Model file for the job. Use its own axes, mm. Face numbers are marked on the shaded views. A direction names the side the tool comes from. Round coordinates to 2 decimals unless told otherwise and drop trailing zeros. Order: outer loops, then holes, each group sorted by start corner. A loop starts at its lowest first (then second) coordinate and runs counter-clockwise, first axis right, second up. Notation, with made-up numbers: (53, -19) -> (81, -19) arc R9 ccw to (81, -4) -> close; hole circle Ø11 at (-36.75, -28). An arc over 180 degrees is marked (long way). Use CSV: the item, a comma, the result in double quotes.
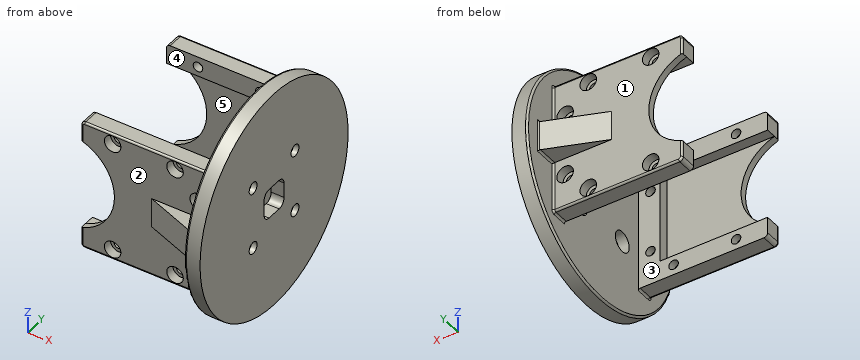
```python
from build123d import *

# Parameters (mm, degrees)
SKETCH1_R           = 1.3
BOSS_EXTRUDE1_DEPTH = 2.8
SKETCH2_R           = 1.3
BOSS_EXTRUDE2_DEPTH = 1.8
SKETCH3_R           = 2.25
CUT_EXTRUDE1_DEPTH  = 2.5
SKETCH4_W           = 35.6
SKETCH4_H           = 4.6
BOSS_EXTRUDE3_DEPTH = 5
SKETCH5_W           = 4.2
SKETCH5_H           = 35.6
BOSS_EXTRUDE4_DEPTH = 15
FILLET1_R           = 1
SKETCH6_R           = 1.6
CUT_EXTRUDE2_DEPTH  = 40.396155741
SKETCH7_R           = 2.8
CUT_EXTRUDE3_DEPTH  = 2.7
CUT_EXTRUDE4_DEPTH  = 3.5
SKETCH9_R           = 30
SKETCH9_W           = 35.6
SKETCH9_H           = 39.2
BOSS_EXTRUDE5_DEPTH = 4.2
BOSS_EXTRUDE6_DEPTH = 4
FILLET2_R           = 0.5
FILLET3_R           = 0.5


with BuildPart() as part:
    # Sketch1 → Boss-Extrude1 (new body)
    with BuildSketch(Plane(origin=(0, 0, 0), x_dir=(1, 0, 0), z_dir=(0, 1, 0))):
        Polygon((33.2, 12.4), (33.2, -12.4), (3.903844259, -12.4), (3.903844259, -17.8), (38.3, -17.8), (38.3, 17.8), (3.903844259, 17.8), (3.903844259, 12.4), align=None)
        with Locations((12.5, 15)):
            Circle(SKETCH1_R, mode=Mode.SUBTRACT)
        with Locations((29.5, 15)):
            Circle(SKETCH1_R, mode=Mode.SUBTRACT)
        with Locations((29.5, -15)):
            Circle(SKETCH1_R, mode=Mode.SUBTRACT)
        with Locations((12.5, -15)):
            Circle(SKETCH1_R, mode=Mode.SUBTRACT)
        with Locations((35.8, -8.5)):
            Circle(SKETCH1_R, mode=Mode.SUBTRACT)
        with Locations((35.8, 8.5)):
            Circle(SKETCH1_R, mode=Mode.SUBTRACT)
    extrude(amount=BOSS_EXTRUDE1_DEPTH)

    # Sketch2 → Boss-Extrude2 (add)
    with BuildSketch(Plane(origin=(0, 2.8, 0), x_dir=(1, 0, 0), z_dir=(0, 1, 0))):
        with BuildLine():
            Line((3.903844259, -12.4), (3.903844259, -17.8))
            Line((3.903844259, -17.8), (38.3, -17.8))
            Line((38.3, -17.8), (38.3, 17.8))
            Line((38.3, 17.8), (3.903844259, 17.8))
            Line((3.903844259, 17.8), (3.903844259, 12.4))
            ThreePointArc((3.903844259, 12.4), (13, 0), (3.903844259, -12.4))
        make_face()
        with Locations((12.5, -15)):
            Circle(SKETCH2_R, mode=Mode.SUBTRACT)
        with Locations((29.5, -15)):
            Circle(SKETCH2_R, mode=Mode.SUBTRACT)
        with Locations((35.8, -8.5)):
            Circle(SKETCH2_R, mode=Mode.SUBTRACT)
        with Locations((35.8, 8.5)):
            Circle(SKETCH2_R, mode=Mode.SUBTRACT)
        with Locations((29.5, 15)):
            Circle(SKETCH2_R, mode=Mode.SUBTRACT)
        with Locations((12.5, 15)):
            Circle(SKETCH2_R, mode=Mode.SUBTRACT)
    extrude(amount=BOSS_EXTRUDE2_DEPTH)

    # Sketch3 → Cut-Extrude1 (cut)
    with BuildSketch(Plane(origin=(0, 4.6, 0), x_dir=(1, 0, 0), z_dir=(0, 1, 0))):
        with Locations((12.5, 15)):
            Circle(SKETCH3_R)
        with Locations((29.5, 15)):
            Circle(SKETCH3_R)
        with Locations((35.8, 8.5)):
            Circle(SKETCH3_R)
        with Locations((35.8, -8.5)):
            Circle(SKETCH3_R)
        with Locations((29.5, -15)):
            Circle(SKETCH3_R)
        with Locations((12.5, -15)):
            Circle(SKETCH3_R)
    extrude(amount=-CUT_EXTRUDE1_DEPTH, mode=Mode.SUBTRACT)

    # Sketch4 → Boss-Extrude3 (add)
    with BuildSketch(Plane(origin=(38.3, 0, 0), x_dir=(0, 0, -1), z_dir=(1, 0, 0))):
        with Locations((0, 2.3)):
            Rectangle(SKETCH4_W, SKETCH4_H)
    extrude(amount=BOSS_EXTRUDE3_DEPTH)

    # Sketch5 → Boss-Extrude4 (add)
    with BuildSketch(Plane.XZ):
        with Locations((41.2, 0)):
            Rectangle(SKETCH5_W, SKETCH5_H)
    extrude(amount=BOSS_EXTRUDE4_DEPTH)

    # Mirror1: part across plane


with BuildPart() as part_1:
    add(part.part)
    add(part.part.mirror(Plane.ZX.offset(-15)))

    # Fillet1
    fillet1_edges = [part_1.edges().sort_by_distance(p)[0] for p in [
        (3.903844259, 2.3, -17.8),
        (3.903844259, 2.3, 17.8),
        (3.903844259, -32.3, 17.8),
        (3.903844259, -32.3, -17.8),
    ]]
    fillet(fillet1_edges, radius=FILLET1_R)

    # Sketch6 → Cut-Extrude2 (cut, through all)
    with BuildSketch(Plane(origin=(43.3, 0, 0), x_dir=(0, 0, -1), z_dir=(1, 0, 0))):
        with Locations((8.485281374, -23.485281374)):
            Circle(SKETCH6_R)
        with Locations((-8.485281374, -23.485281374)):
            Circle(SKETCH6_R)
        with Locations((-8.485281374, -6.514718626)):
            Circle(SKETCH6_R)
        with Locations((8.485281374, -6.514718626)):
            Circle(SKETCH6_R)
    extrude(amount=-CUT_EXTRUDE2_DEPTH, mode=Mode.SUBTRACT)

    # Sketch7 → Cut-Extrude3 (cut)
    with BuildSketch(Plane.ZY.offset(-39.1)):
        with Locations((-8.485281374, -6.514718626)):
            Circle(SKETCH7_R)
        with Locations((8.485281374, -6.514718626)):
            Circle(SKETCH7_R)
        with Locations((-8.485281374, -23.485281374)):
            Circle(SKETCH7_R)
        with Locations((8.485281374, -23.485281374)):
            Circle(SKETCH7_R)
    extrude(amount=-CUT_EXTRUDE3_DEPTH, mode=Mode.SUBTRACT)

    # Sketch8 → Cut-Extrude4 (cut)
    with BuildSketch(Plane(origin=(43.3, 0, 0), x_dir=(0, 0, -1), z_dir=(1, 0, 0))):
        with BuildLine():
            Line((-2.05, -19.05), (2.05, -19.05))
            ThreePointArc((2.05, -19.05), (3.464213562, -18.464213562), (4.05, -17.05))
            Line((4.05, -17.05), (4.05, -12.95))
            ThreePointArc((4.05, -12.95), (3.464213562, -11.535786438), (2.05, -10.95))
            Line((2.05, -10.95), (-2.05, -10.95))
            ThreePointArc((-2.05, -10.95), (-3.464213562, -11.535786438), (-4.05, -12.95))
            Line((-4.05, -12.95), (-4.05, -17.05))
            ThreePointArc((-4.05, -17.05), (-3.464213562, -18.464213562), (-2.05, -19.05))
        make_face()
    extrude(amount=-CUT_EXTRUDE4_DEPTH, mode=Mode.SUBTRACT)

    # Sketch9 → Boss-Extrude5 (add)
    with BuildSketch(Plane(origin=(43.3, 0, 0), x_dir=(0, 0, -1), z_dir=(1, 0, 0))):
        with Locations((0, -15)):
            Circle(SKETCH9_R)
        with Locations((0, -15)):
            Rectangle(SKETCH9_W, SKETCH9_H, mode=Mode.SUBTRACT)
    extrude(amount=-BOSS_EXTRUDE5_DEPTH)

    # Sketch10 → Boss-Extrude6 (add, symmetric)
    with BuildSketch(Plane.XY):
        Polygon((39.1, 10.6), (39.1, 4.6), (23.1, 4.6), align=None)
    boss_extrude6 = extrude(amount=BOSS_EXTRUDE6_DEPTH, both=True)

    # Mirror2: Boss-Extrude6 across plane
    add(boss_extrude6.mirror(Plane(origin=(0, -15, 0), x_dir=(0, 0, 1), z_dir=(0, -1, 0))))

    # Fillet2
    fillet2_edges = [part_1.edges().sort_by_distance(p)[0] for p in [
        (39.1, -15, 30),
    ]]
    fillet(fillet2_edges, radius=FILLET2_R)

    # Fillet3
    fillet3_edges = [part_1.edges().sort_by_distance(p)[0] for p in [
        (3.903844259, -34.6, 14.6),
        (3.903844259, 4.6, -14.6),
        (22.00192213, 4.6, 17.8),
        (4.196737478, 4.6, 17.507106781),
        (4.196737478, 4.6, -17.507106781),
        (3.903844259, -34.6, -14.6),
        (22.00192213, -34.6, 17.8),
        (4.196737478, -34.6, 17.507106781),
        (4.196737478, -34.6, -17.507106781),
        (22.00192213, -34.6, -17.8),
        (22.00192213, 4.6, -17.8),
        (39.1, -32.3, 17.8),
        (39.1, 2.3, 17.8),
        (39.1, -34.6, -10.9),
        (39.1, 2.3, -17.8),
        (39.1, -32.3, -17.8),
        (39.1, 4.6, 10.9),
        (39.1, 4.6, -10.9),
        (39.1, 10.6, 0),
        (39.1, 7.6, -4),
        (39.1, 7.6, 4),
        (39.1, -34.6, 10.9),
        (39.1, -37.6, 4),
        (39.1, -40.6, 0),
        (39.1, -37.6, -4),
        (3.903844259, 4.6, 14.6),
    ]]
    fillet(fillet3_edges, radius=FILLET3_R)


solid = part_1.part
```
Q1. Probe line 1 along X through (y, z) = (3, -15); line 2 along Z through (x, y) = (12.5, -31.2); line 3 along Y through (x, z) = (32, 17). List the from-to ranges inside material, lowest first.
From the geometry:
line 1,"x = 3.9 to 10.25, 14.75 to 27.25, 31.75 to 43.3"
line 2,"z = -17.8 to -16.3, -13.7 to -12.4, 12.4 to 13.7, 16.3 to 17.8"
line 3,"y = -34.6 to -30, 0 to 4.6"
Q2. Which spindle directions (+Z, -Z, +X, -X, +Y, -Y) get a long thin tool onto all of the face, cutting with end or side? Do the marked faces 1, 2 and 3. Say none if no direction does.
From the geometry:
face 1,"-X, +Y"
face 2,"-X, -Y"
face 3,"+Z, -Z, -X"
Q3. Pin check, flat tips, straight feed: pin 1 (1.4 mm diameter, centred on y = -31, z = 2, fed in from -X); pin 2 (1.7 mm diameter, centred on x = 30, y = 8.5, fed in from +Z); pin 3 (7 mm diameter, centred on x = 35.8, z = 8.5, fed in from -Y); pin 4 (2 mm diameter, centred on x = 29.5, y = 3, fed in from -Z). Stop position of each tip, or through.
From the geometry:
pin 1,"stops at x = 33.2"
pin 2,"passes through"
pin 3,"stops at y = -43.8"
pin 4,"stops at z = -17.8"
Q4. Cut at C-C (y = -15). Give the cut face in (x, z).
From the geometry:
outline,"(39.1, -29.5) arc R0.5 ccw to (39.6, -30) -> (43.3, -30) -> (43.3, -4.05) -> (39.8, -4.05) -> (39.8, 4.05) -> (43.3, 4.05) -> (43.3, 30) -> (39.6, 30) arc R0.5 ccw to (39.1, 29.5) -> close"
Q5. Mould opens along Z. For the marked faces 4 and 5 say: +Z half, -Z half, draft (parallel to the pull), parting line (faces both ways), or undercut.
From the geometry:
face 4,"draft"
face 5,"undercut"
Q6. Cut at A-A (x = 17). Give the cut face in (y, z).
From the geometry:
outline,"(-34.6, -17.3) arc R0.5 ccw to (-34.1, -17.8) -> (-30, -17.8) -> (-30, -12.4) -> (-32.8, -12.4) -> (-32.8, 12.4) -> (-30, 12.4) -> (-30, 17.8) -> (-34.1, 17.8) arc R0.5 ccw to (-34.6, 17.3) -> close; (0, -17.8) -> (4.1, -17.8) arc R0.5 ccw to (4.6, -17.3) -> (4.6, 17.3) arc R0.5 ccw to (4.1, 17.8) -> (0, 17.8) -> (0, 12.4) -> (2.8, 12.4) -> (2.8, -12.4) -> (0, -12.4) -> close"
Q7. Cut at D-D (x = 25). Give the cut face in (y, z).
From the geometry:
outline,"(-35.31, -4) -> (-34.6, -4) -> (-34.6, -17.3) arc R0.5 ccw to (-34.1, -17.8) -> (-30, -17.8) -> (-30, -12.4) -> (-32.8, -12.4) -> (-32.8, 12.4) -> (-30, 12.4) -> (-30, 17.8) -> (-34.1, 17.8) arc R0.5 ccw to (-34.6, 17.3) -> (-34.6, 4) -> (-35.31, 4) -> close; (0, -17.8) -> (4.1, -17.8) arc R0.5 ccw to (4.6, -17.3) -> (4.6, -4) -> (5.31, -4) -> (5.31, 4) -> (4.6, 4) -> (4.6, 17.3) arc R0.5 ccw to (4.1, 17.8) -> (0, 17.8) -> (0, 12.4) -> (2.8, 12.4) -> (2.8, -12.4) -> (0, -12.4) -> close"
Q8. Cut at B-B (z = 0). Give the cut face in (x, y).
From the geometry:
outline,"(13, -34.6) -> (23.1, -34.6) -> (38.78, -40.48) arc R0.5 cw to (39.1, -40.95) -> (39.1, -44.5) arc R0.5 ccw to (39.6, -45) -> (43.3, -45) -> (43.3, -19.05) -> (39.8, -19.05) -> (39.8, -10.95) -> (43.3, -10.95) -> (43.3, 15) -> (39.6, 15) arc R0.5 ccw to (39.1, 14.5) -> (39.1, 10.95) arc R0.5 cw to (38.78, 10.48) -> (23.1, 4.6) -> (13, 4.6) -> (13, 2.8) -> (33.2, 2.8) -> (33.2, 0) -> (39.1, 0) -> (39.1, -30) -> (33.2, -30) -> (33.2, -32.8) -> (13, -32.8) -> close"
